Read the model definition and answer for the solid it produces. Units are mm, in the model's axes. A direction names the side the tool comes from. Coordinates: 2 decimals unless noted, no trailing zeros. Order: outer loops, then holes, each group sorted by start corner. A loop starts at its lowest first (then second) coordinate and runs counter-clockwise, first axis right, second up. Notation, with made-up numbers: (45, -39.5) - (62, -39.5) arc R23 ccw to (62, -0.5) - close; hole circle Ø4 at (16.5, 7). An arc over 180 degrees is marked (long way). Use one line per item in the form item = value.
```python
from build123d import *

# Parameters (mm, degrees)
SM_BASE_FLANGE_1_DEPTH = 280
SKETCH_3_R             = 2.5
CUT_EXTRUDE_2_DEPTH    = 327.075144714
CUT_EXTRUDE_3_DEPTH    = 327.075144714
FILLET_1_R             = 5
SKETCH_5_W             = 55
SKETCH_5_H             = 20
CUT_EXTRUDE_4_DEPTH    = 2
EXTRUDE_1_DEPTH        = 55


# Sheet-metal steps are written as plain solids
with BuildPart() as part:
    # Sketch 1 → 基体-法兰1 (new body)
    with BuildSketch(Plane(origin=(0, 0, 0), x_dir=(1, 0, 0), z_dir=(0, 1, 0))):
        with BuildLine():
            Line((105, 63), (15, 63))
            ThreePointArc((15, 63), (4.393398282, 58.606601718), (0, 48))
            Line((0, 48), (0, -48))
            ThreePointArc((0, -48), (4.393398282, -58.606601718), (15, -63))
            Line((15, -63), (105, -63))
            Line((105, -63), (105, -65))
            Line((105, -65), (15, -65))
            ThreePointArc((15, -65), (2.97918472, -60.02081528), (-2, -48))
            Line((-2, -48), (-2, 48))
            ThreePointArc((-2, 48), (2.97918472, 60.02081528), (15, 65))
            Line((15, 65), (105, 65))
            Line((105, 65), (105, 63))
        make_face()
    extrude(amount=SM_BASE_FLANGE_1_DEPTH)

    # 草图3 → 切除-拉伸2 (cut, through all)
    with BuildSketch(Plane.XY.offset(65)):
        with Locations((99.5, 210)):
            Circle(SKETCH_3_R)
        with Locations((99.5, 70)):
            Circle(SKETCH_3_R)
    extrude(amount=-CUT_EXTRUDE_2_DEPTH, mode=Mode.SUBTRACT)

    # 草图4 → 切除-拉伸3 (cut, through all)
    with BuildSketch(Plane.XY.offset(65)):
        Polygon((50, 280), (-2, 228), (-2, 280), align=None)
        Polygon((-2, 52), (-2, 0), (50, 0), align=None)
    extrude(amount=-CUT_EXTRUDE_3_DEPTH, mode=Mode.SUBTRACT)

    # 圆角1
    fillet_1_edges = [part.edges().sort_by_distance(p)[0] for p in [
        (105, 0, 64),
        (105, 0, -64),
        (105, 280, 64),
        (105, 280, -64),
    ]]
    fillet(fillet_1_edges, radius=FILLET_1_R)

    # 草图5 → 切除-拉伸4 (cut)
    with BuildSketch(Plane(origin=(0, 0, -65), x_dir=(-1, 0, 0), z_dir=(0, 0, -1))):
        with Locations((-77.5, 86)):
            Rectangle(SKETCH_5_W, SKETCH_5_H)
    extrude(amount=-CUT_EXTRUDE_4_DEPTH, mode=Mode.SUBTRACT)

    # 草图6 → 凸台-拉伸1 (add)
    with BuildSketch(Plane(origin=(50, 0, 0), x_dir=(0, 0, -1), z_dir=(1, 0, 0))):
        Polygon((65, 96), (80, 96), (80, 76), (65, 76), (65, 74), (82, 74), (82, 98), (65, 98), align=None)
    extrude(amount=EXTRUDE_1_DEPTH)


solid = part.part
```
(1) Section A-A, the plane y = 30 is taken. Write down the section's boundary in (x, z).
Answer list:
outline = (20, -65) - (105, -65) - (105, -63) - (20, -63) - close; (20, 63) - (105, 63) - (105, 65) - (20, 65) - close
(2) Given pin 1 Ø6 at (x, y) = (99.5, 210) entering from -Z; pin 2 Ø1.6 at (y, z) = (85, -63.5) entering from +X; pin 3 Ø12 at (y, z) = (68, -45.5) entering from +X, each flat-ended and moving along its own axis, determine where each tip first touches the part or whether it passes through.
Answer list:
pin_1 = -65
pin_2 = 50
pin_3 = 0.41
(3) Which of the six approach directions +Z, -Z, +X, -X, +Y, -Y give full straight-line access (tool end or side, diameter ignored) to faces 4 (the flat face through (77, 86, -80)), 5 (the flat face through (77, 74, -73)), 6 (the flat face through (77, 86, -82)), 7 (the cylindrical face through (4.28, 138.53, 58.49)), 8 (the flat face through (77, 98, -74))?
Answer list:
face_4 = +X, -X
face_5 = -Z, +X, -X, -Y
face_6 = -Z, +X, -X, +Y, -Y
face_7 = +X, +Y, -Y
face_8 = -Z, +X, -X, +Y
(4) Section B-B, the plane x = 23 is taken. Write down the section's boundary in (y, z), then the cut area to 3 significant figures.
Answer list:
outline = (27, -65) - (253, -65) - (253, -63) - (27, -63) - close; (27, 63) - (253, 63) - (253, 65) - (27, 65) - close
area = 904 mm2
(5) Section D-D, the plane x = 64.5 is taken. Write down the section's boundary in (y, z).
Answer list:
outline = (0, -65) - (74, -65) - (74, -82) - (98, -82) - (98, -65) - (280, -65) - (280, -63) - (96, -63) - (96, -80) - (76, -80) - (76, -63) - (0, -63) - close; (0, 63) - (280, 63) - (280, 65) - (0, 65) - close
(6) Section C-C, the plane y = 88 is taken. Write down the section's boundary in (x, z), then the cut area to 3 significant figures.
Answer list:
outline = (-2, -48) arc R17 ccw to (15, -65) - (50, -65) - (50, -63) - (15, -63) arc R15 cw to (0, -48) - (0, 48) arc R15 cw to (15, 63) - (105, 63) - (105, 65) - (15, 65) arc R17 ccw to (-2, 48) - close; (50, -82) - (105, -82) - (105, -80) - (50, -80) - close
area = 653 mm2
(7) Straight lines are drawn through the part: L1, parallel to Y at x = 99.5, z = -63.35; L2, parallel to Z at x = 79, y = 78; L3, parallel to Z at x = 84.5, y = 105. For each, find the intervals that lie inside material, in ascending order.
Answer list:
L1 = 0 to 67.5, 72.5 to 76, 96 to 207.5, 212.5 to 280
L2 = -82 to -80, 63 to 65
L3 = -65 to -63, 63 to 65
(8) The mould has two halves that part along Y. Classify faces 1 (the flat face through (77, 96, -71)), 2 (the flat face through (-2, 139, 1)), 3 (the flat face through (-1, 229, 0)): +Y half, -Y half, draft (parallel to the pull), parting line (faces both ways), or undercut.
Answer list:
face_1 = undercut
face_2 = draft
face_3 = +Y half
